Geometry check sheet. Reference: the model listing, model coordinates, mm. A direction names the side the tool comes from. Round coordinates to 2 decimals unless told otherwise and drop trailing zeros. Write each loop counter-clockwise with the first axis right and the second up, starting at its lowest first coordinate (ties: lowest second). Pieces come first, ordered by that corner, then holes.
Item 1: Depth check by flat-ended pin: P1, Ø5, axis at x = 237.5, z = 396, coming from the -Y side; P2, Ø1, axis at y = 37.5, z = 357, coming from the +X side; P3, Ø6, axis at x = 246, z = 372, coming from the -Y side. Enter the tip coordinate at first touch or a pass-through.
Item 2: Cross-section at B-B (z = 339). Enter the section's corners in (x, y).
Item 3: Scan lines: probe 1 along Y at (x, z) = (240.25, 397.5); probe 2 along Y at (x, z) = (239.75, 397); probe 3 along Z at (x, y) = (240.5, -3). Record each from-to range of solid material in increasing order.
Item 4: Access from +Z, -Z, +X, -X, +Y, -Y to the whole of each face (thin tool, end or side, straight path). Record for faces 1 (the face through (234.1, -39.6, 357)), 2 (the face through (240, 45, 323)).
Item 5: Draft check along Y on faces 3 (the face through (238.959, 0.294, 406.068)), 4 (the face through (240, -45, 323)). Enter one of: pulls with the +Y half, pulls with the -Y half, needs draft (parallel to the pull), parting line crosses it, or undercut.
Item 6: Cross-section at A-A (x = 240). Enter the section's corners in (y, z), then the cut area to 3 significant figures.
from build123d import *

# Parameters (mm, degrees)
PIPE_1_PROFILE_R = 8


with BuildPart() as part:
    # Pipe 1: sweep along a curve in space
    with BuildLine() as pipe_1_path:
        Line((240, -45, 323), (240, -45, 390))
        ThreePointArc((240, -45, 390), (240, -37.970562748, 406.970562748), (240, -21, 414))
        Line((240, -21, 414), (240, 21, 414))
        ThreePointArc((240, 21, 414), (240, 37.970562748, 406.970562748), (240, 45, 390))
        Line((240, 45, 390), (240, 45, 323))
    # Pipe 1 profile (on start of the path) → Pipe 1 (sweep)
    with BuildSketch(Plane(origin=(240, -45, 323), x_dir=(1, 0, 0), z_dir=(0, 0, 1))):
        Circle(PIPE_1_PROFILE_R)
    sweep(path=pipe_1_path.line)


solid = part.part
Resolved:
1. P1: stops at y = -52.69
1. P2: stops at x = 243.87
1. P3: stops at y = -52.42
2. outline: circle Ø16 at (240, -45); circle Ø16 at (240, 45)
3. probe 1: y = -52.1 to -35.14, 35.14 to 52.1
3. probe 2: y = -52.22 to -35.39, 35.39 to 52.22
3. probe 3: z = 406.02 to 421.98
4. face 1: -Z
4. face 2: -Z, +X, -X, +Y, -Y
5. face 3: undercut
5. face 4: needs draft
6. outline: (-53, 323) - (-37, 323) - (-37, 390) arc R16 cw to (-21, 406) - (21, 406) arc R16 cw to (37, 390) - (37, 323) - (53, 323) - (53, 390) arc R32 ccw to (21, 422) - (-21, 422) arc R32 ccw to (-53, 390) - close
6. area: 4,020 mm2
